For this review, use the dimensioned drawing (mm, ordinates from the lowest corner) and the shaded views. A direction names the side the tool comes from. Coordinates: 2 decimals unless noted, no trailing zeros. Order: outer loops, then holes, each group sorted by start corner. A loop starts at its lowest first (then second) coordinate and runs counter-clockwise, first axis right, second up. Notation, with made-up numbers: M -12,29 L 44,29 A27 cw 44,45 Z; hole C 14,63 d10. An arc over 180 degrees is marked long. Use one line per item in the form item = value. Start each with the question number.
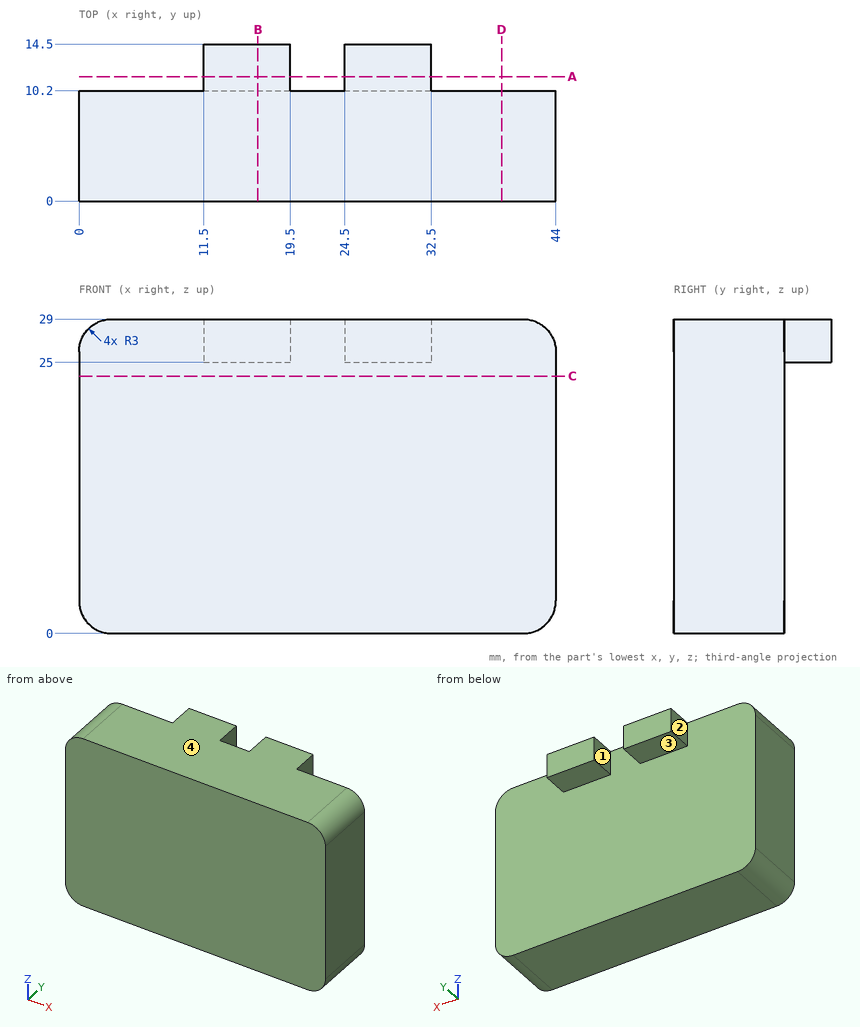
1. Tool access review of the marked faces 1, 2, 3 and 4: name each direction out of +Z, -Z, +X, -X, +Y, -Y from which nothing blocks a thin tool from reaching the whole face with its end or side.
2. Consider section D-D, the plane x = 39. Write out the cut boundary in (y, z), plus the area to 3 significant figures.
3. For pin 1 Ø3 at (y, z) = (11.5, 28) entering from -X; pin 2 Ø2 at (x, y) = (21.5, 12.5) entering from -Z; pin 3 Ø4.5 at (y, z) = (13, 26.5) entering from +X; pin 4 Ø1.3 at (x, y) = (27, 12) entering from -Z, all flat-tipped, find the tip position at first contact; note any pin that passes through.
4. Consider section C-C, the plane z = 23.75. Write out the cut boundary in (x, y).
5. Consider section B-B, the plane x = 16.5. Write out the cut boundary in (y, z), plus the area to 3 significant figures.
6. Consider section A-A, the plane y = 11.5. Write out the cut boundary in (x, z), plus the area to 3 significant figures.
7. To check wall thickness, follow line 1 (Y direction, x = 2, z = 13.75). State the ranges of the line that lie inside material, in increasing order.
Answers follow:
q1.face_1 = +Z, -Z, +Y
q1.face_2 = +Z, -Z, -X, +Y
q1.face_3 = -Z, +X, -X, +Y
q1.face_4 = +Z, +X, -X, +Y, -Y
q2.outline = M 0,0 L 10.2,0 L 10.2,29 L 0,29 Z
q2.area = 296 mm²
q3.pin_1 = 0.27
q3.pin_2 = through
q3.pin_3 = 32.5
q3.pin_4 = 25
q4.outline = M 0,0 L 44,0 L 44,10.2 L 0,10.2 Z
q5.outline = M 0,0 L 10.2,0 L 10.2,25 L 14.5,25 L 14.5,29 L 0,29 Z
q5.area = 313 mm²
q6.outline = M 11.5,25 L 19.5,25 L 19.5,29 L 11.5,29 Z; M 24.5,25 L 32.5,25 L 32.5,29 L 24.5,29 Z
q6.area = 64.0 mm²
q7.line_1 = 0 to 10.2
